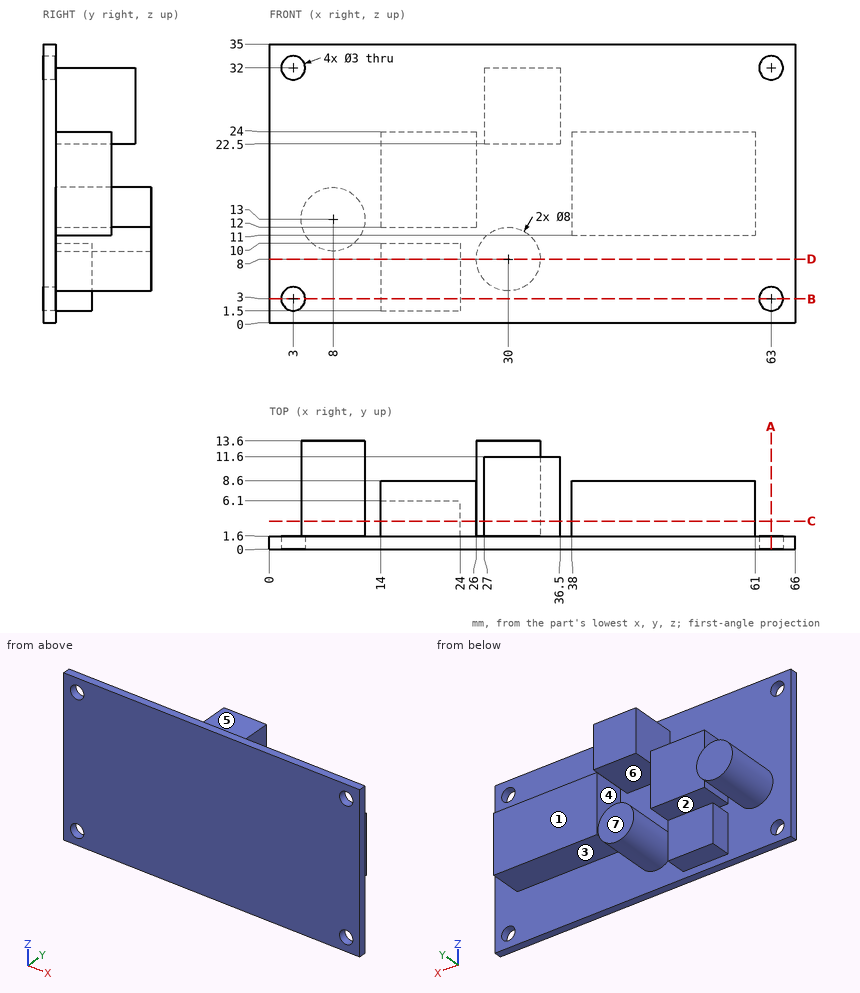
Drawing for the job (mm, zero at the part's lowest x, y, z). A direction names the side the tool comes from. Round coordinates to 2 decimals unless told otherwise and drop trailing zeros. Loops run counter-clockwise (first coordinate to the right, second up) from the corner with the lowest first, then second, coordinate; pieces in that order, holes last. Notation, with made-up numbers: M 68,7.5 L 110,7.5 A22 ccw 110,32.5 Z; hole C -12.75,-33 d9. An arc over 180 degrees is marked long. Use a Markdown table: item, result. Add a question column.
(1) Which spindle directions (+Z, -Z, +X, -X, +Y, -Y) get a long thin tool onto all of the face, cutting with end or side? Do the marked faces 1, 2, 3, 4 and 5. Say none if no direction does.
(2) Pull direction X, two halves, no side cores. Call the marked faces 6 and 7: +X half, -X half, draft (parallel to the pull), parting line (faces both ways), or undercut.
(3) Drill centre lines: line 1 (X direction, y = 0.8, z = 3); line 2 (Z direction, x = 3, y = 0.45); line 3 (X direction, y = 2, z = 21.5). Where is each one in solid material? Low to high.
(4) Flat gauge pins, fed straight in: pin 1 (8 mm diameter, centred on y = 6, z = 23.5, fed in from -X); pin 2 (1.5 mm diameter, centred on y = 3.5, z = 24, fed in from +X); pin 3 (2 mm diameter, centred on x = 22.5, y = 5, fed in from +Z). Where does each tip first touch, or does it go through?
(5) Cut at A-A (x = 63). Give the cut face in (y, z).
(6) Cut at D-D (z = 8). Give the cut face in (x, y), and give its area (3 significant figures).
(7) Cut at C-C (y = 3.5). Give the cut face in (x, z).
(8) Cut at B-B (z = 3). Give the cut face in (x, y), and give its area (3 significant figures).
Geometry says:
| question | item | result |
|---|---|---|
| 1 | face 1 | +Z, -Z, +X, +Y |
| 1 | face 2 | +Y |
| 1 | face 3 | -Z, +X, +Y |
| 1 | face 4 | +Z, -Z, +Y |
| 1 | face 5 | +Z, +X, -X, +Y |
| 2 | face 6 | undercut |
| 2 | face 7 | draft |
| 3 | line 1 | x = 0 to 1.5, 4.5 to 61.5, 64.5 to 66 |
| 3 | line 2 | z = 0 to 1.5, 4.5 to 30.5, 33.5 to 35 |
| 3 | line 3 | x = 14 to 26, 38 to 61 |
| 4 | pin 1 | stops at x = 14 |
| 4 | pin 2 | stops at x = 61 |
| 4 | pin 3 | stops at z = 24 |
| 5 | outline | M 0,0 L 1.6,0 L 1.6,1.5 L 0,1.5 Z; M 0,4.5 L 1.6,4.5 L 1.6,30.5 L 0,30.5 Z; M 0,33.5 L 1.6,33.5 L 1.6,35 L 0,35 Z |
| 6 | outline | M 0,0 L 66,0 L 66,1.6 L 34,1.6 L 34,13.6 L 26,13.6 L 26,1.6 L 24,1.6 L 24,6.1 L 14,6.1 L 14,1.6 L 0,1.6 Z |
| 6 | area | 247 mm² |
| 7 | outline | C 8,13 d8; M 14,1.5 L 24,1.5 L 24,10 L 14,10 Z; M 14,12 L 26,12 L 26,24 L 14,24 Z; C 30,8 d8; M 27,22.5 L 36.5,22.5 L 36.5,32 L 27,32 Z; M 38,11 L 61,11 L 61,24 L 38,24 Z |
| 8 | outline | M 0,0 L 1.5,0 L 1.5,1.6 L 0,1.6 Z; M 4.5,0 L 61.5,0 L 61.5,1.6 L 24,1.6 L 24,6.1 L 14,6.1 L 14,1.6 L 4.5,1.6 Z; M 64.5,0 L 66,0 L 66,1.6 L 64.5,1.6 Z |
| 8 | area | 141 mm² |
